from build123d import *

# Parameters (mm, degrees)
F0_W     = 25
F0_H     = 600
F1_DEPTH = 25
F2_R     = 12.49999
F3_R     = 12.49999
F4_R     = 5
F5_DEPTH = 25


# Not quite as in the source:
# - a fillet or chamfer is up to 0.001 mm smaller than in the source, because OpenCascade refuses the exact size
# - a pattern or mirror of a feature is missing from the dataset's text; its kind, count and spacing are read off the source's solid


with BuildPart() as f1:
    # F0 (on Front) → F1 (new body)
    with BuildSketch(Plane.XZ):
        Rectangle(F0_W, F0_H)
    extrude(amount=F1_DEPTH)

    # F2 (radius 12.5 in the source; OpenCascade refuses exactly that, so slightly less here)
    f2_edges = [f1.edges().sort_by_distance(p)[0] for p in [
        (-12.5, -12.5, 300),
        (12.5, -12.5, 300),
    ]]
    fillet(f2_edges, radius=F2_R)

    # F3 (radius 12.5 in the source; OpenCascade refuses exactly that, so slightly less here)
    f3_edges = [f1.edges().sort_by_distance(p)[0] for p in [
        (-12.5, -12.5, -300),
        (12.5, -12.5, -300),
    ]]
    fillet(f3_edges, radius=F3_R)

    # F4 (on face) → F5 (cut)
    with BuildSketch(Plane.XZ.offset(25)):
        with Locations((0, 287.5)):
            Circle(F4_R)
    f5 = extrude(amount=-F5_DEPTH, mode=Mode.SUBTRACT)

    # F5_copies: F5 across plane
    add(f5.mirror(Plane(origin=(0, 0, 0), x_dir=(-1, 0, 0), z_dir=(0, 0, -1))), mode=Mode.SUBTRACT)


solid = f1.part
CAD build for the part. Positions are in the model's coordinates, mm. Give positions to 0.01 mm unless a question says otherwise; leave off trailing zeros. Write each question's results on one line, items separated by ' | '.
1. Probe L1, parallel to Z at x = -0.25, y = -11.5; L2, parallel to X at y = -6.5, z = -287.5; L3, parallel to Z at x = 11.5, y = -14.75. List the from-to ranges inside material, lowest first. Write a range as from..to.
Calculated:
L1: z = -300..-292.49, -282.51..282.51, 292.49..300 | L2: x = -12.5..-5, 5..12.5 | L3: z = -292.4..292.4
2. Saw through at A-A on y = -5.5. Count the separate pieces of the cut face and the enclosed holes in it, and give its area (3 significant figures).
Calculated:
separate pieces: 1 | enclosed holes: 2 | area: 14,700 mm2
3. Pull direction Z, two halves, no side cores. Call faces 1 (the face through (-0.651, -12.675, 292.457)), 2 (the face through (0, -25, 4)), 3 (the face through (8.935, -12.675, 296.241)): released by +Z, released by -Z, zero draft, split by the parting line, or undercut.
Calculated:
face 1: undercut | face 2: zero draft | face 3: released by +Z
4. Pin check, flat tips, straight feed: pin 1 (2 mm diameter, centred on x = -8, y = -2.5, fed in from +Z); pin 2 (1.5 mm diameter, centred on x = 3.5, y = -11, fed in from -Z); pin 3 (4 mm diameter, centred on x = -9.5, z = -239, fed in from +Y). Stop position of each tip, or through.
Calculated:
pin 1: stops at z = 297.86 | pin 2: stops at z = -299.69 | pin 3: stops at y = 0
